Geometry check sheet. Reference: drawing and pictorial views, mm from the part's lowest x, y, z. Give positions to 0.01 mm unless a question says otherwise; leave off trailing zeros. Write each loop counter-clockwise with the first axis right and the second up, starting at its lowest first coordinate (ties: lowest second). Pieces come first, ordered by that corner, then holes. Notation, with made-up numbers: M -35.75,78 L -29.75,78 A16 ccw -29.75,108 Z; hole C 12.25,-28 d5. An arc over 180 degrees is marked long. One line per item, written item: value. Start each with the question number.
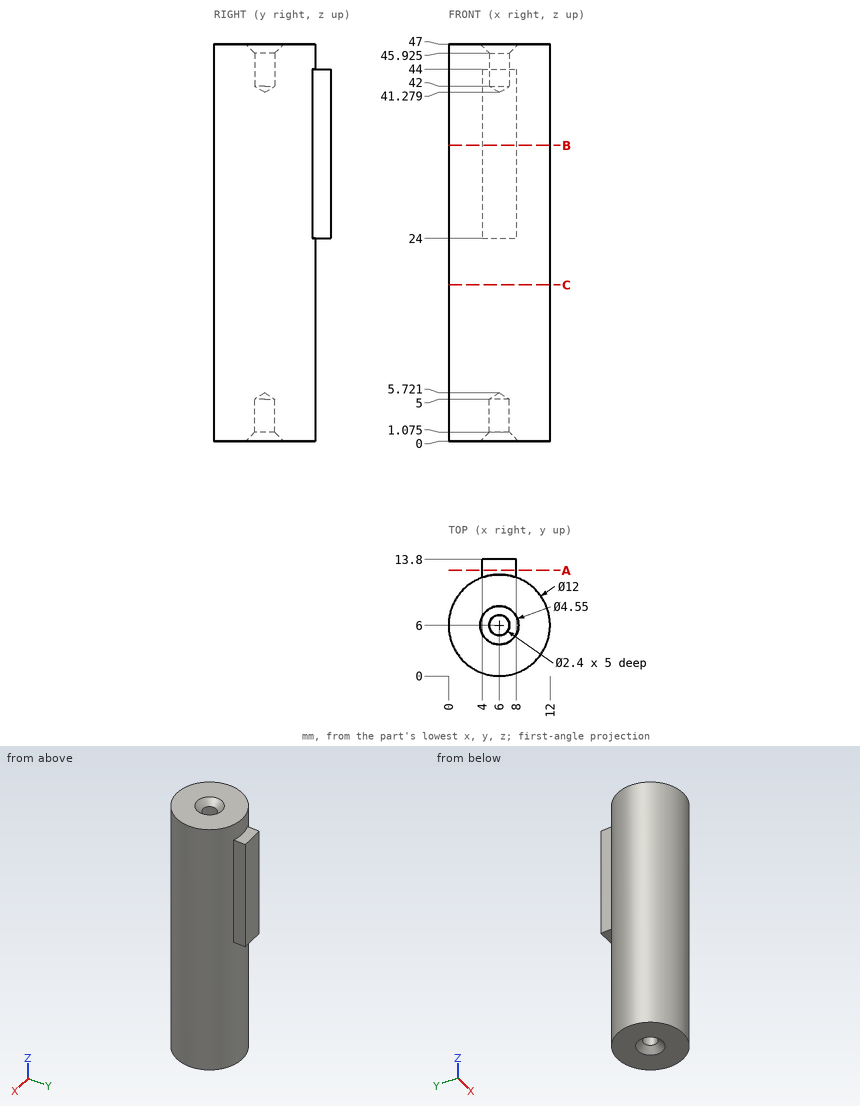
1) Gauge pin test, flat ends, axial feed: pin 1 (1.1 mm diameter, centred on y = 13, z = 35, fed in from -X); pin 2 (1.9 mm diameter, centred on x = 6, y = 6, fed in from +Z); pin 3 (8 mm diameter, centred on y = 10.5, z = 12, fed in from -X). Record the tip position at first contact, or that the pin passes through.
2) Cross-section at C-C (z = 18.5). Record the boundary of the cut face in (x, y).
3) Material ranges on L1, parallel to Y at x = 6, z = 43.55; L2, parallel to Y at x = 6, z = 44.55; L3, parallel to X at y = 12, z = 41, recorded low to high. Write a range as from..to.
4) Cross-section at A-A (y = 12.5). Record the boundary of the cut face in (x, z), plus the area to 3 significant figures.
5) Cross-section at B-B (z = 35). Record the boundary of the cut face in (x, y), plus the area to 3 significant figures.
Data:
1. pin 1: stops at x = 4
1. pin 2: stops at z = 41.85
1. pin 3: stops at x = 0.02
2. outline: C 6,6 d12
3. L1: y = 0..4.8, 7.2..13.8
3. L2: y = 0..4.8, 7.2..12
3. L3: x = 4..8
4. outline: M 4,24 L 8,24 L 8,44 L 4,44 Z
4. area: 80.0 mm2
5. outline: M 4,11.66 A6 ccw long 8,11.66 L 8,13.8 L 4,13.8 Z
5. area: 121 mm2
